Print and shaded views of the part. All mm, measured from the part's lowest x, y and z. A direction names the side the tool comes from. Give positions to 0.01 mm unless a question says otherwise; leave off trailing zeros. Order: outer loops, then holes, each group sorted by start corner. A loop starts at its lowest first (then second) coordinate and runs counter-clockwise, first axis right, second up. Notation, with made-up numbers: (22.5, 65.25) - (74.5, 65.25) arc R14 ccw to (74.5, 91.25) - close; hole circle Ø9 at (-6.5, 71.5). An arc over 180 degrees is marked (long way). Answer in a Markdown table with one row per item.
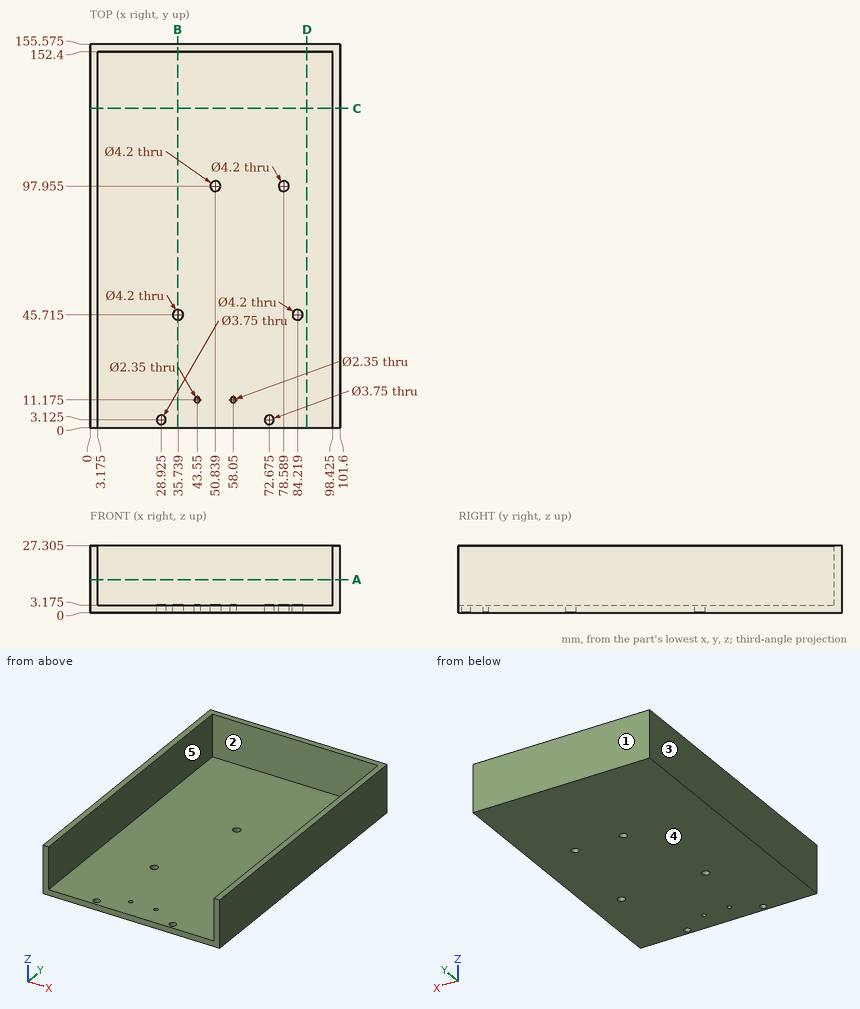
1. Cut at D-D on x = 88. Write the cut outline in (y, z) (1 decimal).
Check result:
| item | result |
|---|---|
| outline | (0, 0) - (155.6, 0) - (155.6, 27.3) - (152.4, 27.3) - (152.4, 3.2) - (0, 3.2) - close |
2. Drop flat-ended pins along their axis: P1, Ø10, axis at x = 27, y = 49, coming from the -Z side; P2, Ø6, axis at x = 90.5, y = 97.5, coming from the +Z side (3 decimals). Give the stop position or say it passes through.
Check result:
| item | result |
|---|---|
| P1 | stops at z = 0 |
| P2 | stops at z = 3.175 |
3. Probe line 1 (X direction, y = 147, z = 9.25) (1 decimal); line 2 (Z direction, x = 81, y = 94.5) (1 decimal); line 3 (Y direction, x = 52, z = 17.25) (1 decimal). List the from-to ranges inside material, lowest first.
Check result:
| item | result |
|---|---|
| line 1 | x = 0 to 3.2, 98.4 to 101.6 |
| line 2 | z = 0 to 3.2 |
| line 3 | y = 152.4 to 155.6 |
4. Two-plate mould, pull along X, no slides. Class the marked faces 1, 2 and 3: +X half, -X half, draft (parallel to the pull), parting line (faces both ways), or undercut.
Check result:
| item | result |
|---|---|
| face 1 | draft |
| face 2 | undercut |
| face 3 | -X half |
5. Cut at A-A on z = 13.5. Write the cut outline in (x, y) (1 decimal), and give its area (3 significant figures).
Check result:
| item | result |
|---|---|
| outline | (0, 0) - (3.2, 0) - (3.2, 152.4) - (98.4, 152.4) - (98.4, 0) - (101.6, 0) - (101.6, 155.6) - (0, 155.6) - close |
| area | 1,290 mm² |
6. Cut at B-B on x = 35.5. Write the cut outline in (y, z) (1 decimal).
Check result:
| item | result |
|---|---|
| outline | (0, 0) - (43.6, 0) - (43.6, 3.2) - (0, 3.2) - close; (47.8, 0) - (155.6, 0) - (155.6, 27.3) - (152.4, 27.3) - (152.4, 3.2) - (47.8, 3.2) - close |
7. Which spindle directions (+Z, -Z, +X, -X, +Y, -Y) get a long thin tool onto all of the face, cutting with end or side? Do the marked faces 4 and 5. Say none if no direction does.
Check result:
| item | result |
|---|---|
| face 4 | -Z, +X, -X, +Y, -Y |
| face 5 | +Z, -Y |
8. Cut at C-C on y = 129.5. Write the cut outline in (x, z) (1 decimal).
Check result:
| item | result |
|---|---|
| outline | (0, 0) - (101.6, 0) - (101.6, 27.3) - (98.4, 27.3) - (98.4, 3.2) - (3.2, 3.2) - (3.2, 27.3) - (0, 27.3) - close |
